```python
from build123d import *

# Parameters (mm, degrees)
F0_W     = 7.1
F0_H     = 7.1
F1_DEPTH = 25
F2_R     = 0.75
F3_DEPTH = 25
F4_R     = 0.5
F5_DEPTH = 5


with BuildPart() as f1:
    # F0 (on Front) → F1 (new body)
    with BuildSketch(Plane.XZ):
        with Locations((22.369518, -20.953149)):
            Rectangle(F0_W, F0_H)
    extrude(amount=F1_DEPTH)

    # F2 (on face) → F3 (cut)
    with BuildSketch(Plane(origin=(0, 0, -24.503149), x_dir=(1, 0, 0), z_dir=(0, 0, -1))):
        with Locations((22.369518, 23)):
            Circle(F2_R)
    extrude(amount=-F3_DEPTH, mode=Mode.SUBTRACT)

    # F4 (on face) → F5 (cut)
    with BuildSketch(Plane(origin=(0, 0, 0), x_dir=(-1, 0, 0), z_dir=(0, 1, 0))):
        with Locations((-22.369518, -20.953149)):
            Circle(F4_R)
    extrude(amount=-F5_DEPTH, mode=Mode.SUBTRACT)


solid = f1.part
```
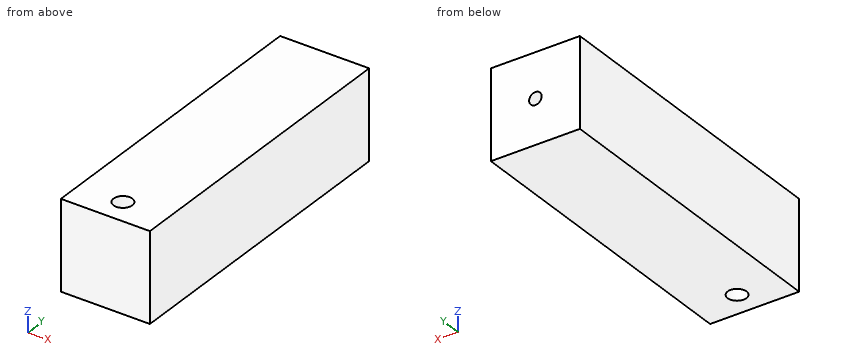
CAD build for the part. Positions are in the model's coordinates, mm. Coordinates: 2 decimals unless noted, no trailing zeros. Write each loop counter-clockwise with the first axis right and the second up, starting at its lowest first coordinate (ties: lowest second). Pieces come first, ordered by that corner, then holes. Notation, with made-up numbers: (62.25, 29) -> (109.25, 29) arc R37 cw to (109.25, 66) -> close; hole circle Ø9 at (-6.5, -21.5). An arc over 180 degrees is marked (long way). Use CSV: the item, a comma, the result in double quotes. Start each with the question number.
Item 1: Band-saw the part on B-B, the plane x = 22.25. Write the cut outline in (y, z), plus the area to 3 significant figures.
Item 2: Drop a flat-ended pin along its axis: P1, Ø0.8, axis at x = 22.5, z = -21, coming from the +Y side. Give the stop position or say it passes through.
Item 3: Band-saw the part on A-A, the plane y = -23. Write the cut outline in (x, z), plus the area to 3 significant figures.
Item 4: Wall check: probe 1 along X at (y, z) = (-23, -20.75); probe 2 along X at (y, z) = (-4.25, -21); probe 3 along Y at (x, z) = (23, -18.25). Give the ranges that are in metal, low to high.
Response values:
1,outline,"(-25, -24.5) -> (-23.74, -24.5) -> (-23.74, -17.4) -> (-25, -17.4) -> close; (-22.26, -24.5) -> (0, -24.5) -> (0, -21.44) -> (-5, -21.44) -> (-5, -20.47) -> (0, -20.47) -> (0, -17.4) -> (-22.26, -17.4) -> close"
1,area,"162 mm2"
2,P1,"stops at y = 0"
3,outline,"(18.82, -24.5) -> (21.62, -24.5) -> (21.62, -17.4) -> (18.82, -17.4) -> close; (23.12, -24.5) -> (25.92, -24.5) -> (25.92, -17.4) -> (23.12, -17.4) -> close"
3,area,"39.8 mm2"
4,probe 1,"x = 18.82 to 21.62, 23.12 to 25.92"
4,probe 2,"x = 18.82 to 21.87, 22.87 to 25.92"
4,probe 3,"y = -25 to -23.41, -22.59 to 0"
